```python
from build123d import *

# Parameters (mm, degrees)
FILLET1_R                          = 1.27
SKETCH3_R                          = 39.37
SKETCH3_R_2                        = 11.43
CUT_EXTRUDE1_DEPTH                 = 6.35
CHAMFER1_SIZE                      = 1.27
FILLET2_R                          = 1.27
F_3_16_0_1875_DIAMETER_HOLE1_D     = 4.7625
F_3_16_0_1875_DIAMETER_HOLE1_DEPTH = 13.97
F_3_16_0_1875_DIAMETER_HOLE1_TIP   = 1.430799349


with BuildPart() as part:
    # Sketch1 → Revolve1 (revolve)
    with BuildSketch(Plane.XY):
        Polygon((-17.49338415, -39.37), (-17.49338415, -50.8), (-14.31838415, -50.8), (-14.31838415, -39.37), (5.36661585, -39.37), (5.36661585, -8.89), (0.104252055, -8.89), align=None)
    revolve(axis=Axis((18.935801868, 0, 0), (-1, 0, 0)))

    # Fillet1
    fillet1_edges = [part.edges().sort_by_distance(p)[0] for p in [
        (-14.31838415, 39.37, 0),
    ]]
    fillet(fillet1_edges, radius=FILLET1_R)

    # Sketch3 → Cut-Extrude1 (cut)
    with BuildSketch(Plane(origin=(5.36661585, 0, 0), x_dir=(0, 0, -1), z_dir=(1, 0, 0))):
        Circle(SKETCH3_R)
        Circle(SKETCH3_R_2, mode=Mode.SUBTRACT)
    extrude(amount=-CUT_EXTRUDE1_DEPTH, mode=Mode.SUBTRACT)

    # Chamfer1
    chamfer1_edges = [part.edges().sort_by_distance(p)[0] for p in [
        (-0.98338415, 39.37, 0),
        (-14.31838415, 50.8, 0),
    ]]
    chamfer(chamfer1_edges, length=CHAMFER1_SIZE)

    # Fillet2
    fillet2_edges = [part.edges().sort_by_distance(p)[0] for p in [
        (-0.98338415, 0, 11.43),
    ]]
    fillet(fillet2_edges, radius=FILLET2_R)

    # 3/16 (0.1875) Diameter Hole1
    with Locations(Plane.ZY.offset(17.49338415)):
        with Locations((-44.45, 0), (0, 44.45), (44.45, 0), (0, -44.45)):
            Hole(F_3_16_0_1875_DIAMETER_HOLE1_D / 2, depth=F_3_16_0_1875_DIAMETER_HOLE1_DEPTH)
            with Locations((0, 0, -(F_3_16_0_1875_DIAMETER_HOLE1_DEPTH + F_3_16_0_1875_DIAMETER_HOLE1_TIP / 2))):  # 118° drill point
                Cone(0, F_3_16_0_1875_DIAMETER_HOLE1_D / 2, F_3_16_0_1875_DIAMETER_HOLE1_TIP, mode=Mode.SUBTRACT)


solid = part.part
```
For this review, take the finished solid that the model builds, in its own axes (mm). A direction names the side the tool comes from. Round coordinates to 2 decimals unless told otherwise and drop trailing zeros. Write each loop counter-clockwise with the first axis right and the second up, starting at its lowest first coordinate (ties: lowest second). Pieces come first, ordered by that corner, then holes.
1) Insertion check: pin 1 Ø1.5 at (x, y) = (-3, 22) entering from +Z; pin 2 Ø8 at (x, y) = (-2, -36.5) entering from -Z; pin 3 Ø10 at (x, z) = (-8.5, 38.5) entering from -Y; pin 4 Ø4.5 at (y, z) = (0, -44.45) entering from +X. Each pin has a flat end and moves straight along its axis. Give the tip position at first contact, or say it passes through.
Answer below:
pin 1: stops at z = 33.14
pin 2: stops at z = -22.21
pin 3: stops at y = -20.68
pin 4: passes through
2) Machinability: for faces 1 (the face through (-14.318, 18.6, -36.5)), 2 (the face through (-17.493, -38, 12)), which of the approach directions +Z, -Z, +X, -X, +Y, -Y give a long, thin tool a straight path to every point of the face, cutting with its end or side? Answer none if there is none.
Answer below:
face 1: +X
face 2: +Z, -Z, -X, +Y, -Y
3) For line 1 along Z through (x, y) = (3.5, -1); line 2 along Z through (x, y) = (-9.5, -0.5); line 3 along X through (y, z) = (23, 41.5), list the stretches that pass through material, from the lowest coordinate up.
Answer below:
line 1: z = -11.39 to -8.83, 8.83 to 11.39
line 2: z = -39.37 to -25.52, 25.52 to 39.37
line 3: x = -17.49 to -14.32
4) Mouldability with a two-part tool opening along Y and no side actions: class faces 3 (the face through (-16.528, 11.012, -49.592)), 4 (the face through (5.367, -6, -7)), 5 (the face through (-15.88, 0.1, 46.83)) as +Y half, -Y half, draft (parallel to the pull), parting line (faces both ways), or undercut.
Answer below:
face 3: parting line
face 4: draft
face 5: undercut
5) Take a section at A-A on y = 0. State how many separate pieces and enclosed holes the cut face has, then the cut area to 3 significant figures.
Answer below:
separate pieces: 4
enclosed holes: 0
area: 543 mm2
6) Take a section at B-B on x = -7.25. Give the boundary of the cut face in (y, z), then the cut area to 3 significant figures.
Answer below:
outline: circle Ø78.74 at (0, 0); hole circle Ø43.26 at (0, 0)
area: 3,400 mm2
